Check sheet for the drawn part. Datum: minimum x, y, z corner. Units: mm. Give positions to 0.01 mm unless a question says otherwise; leave off trailing zeros. Loops run counter-clockwise (first coordinate to the right, second up) from the corner with the lowest first, then second, coordinate; pieces in that order, holes last.
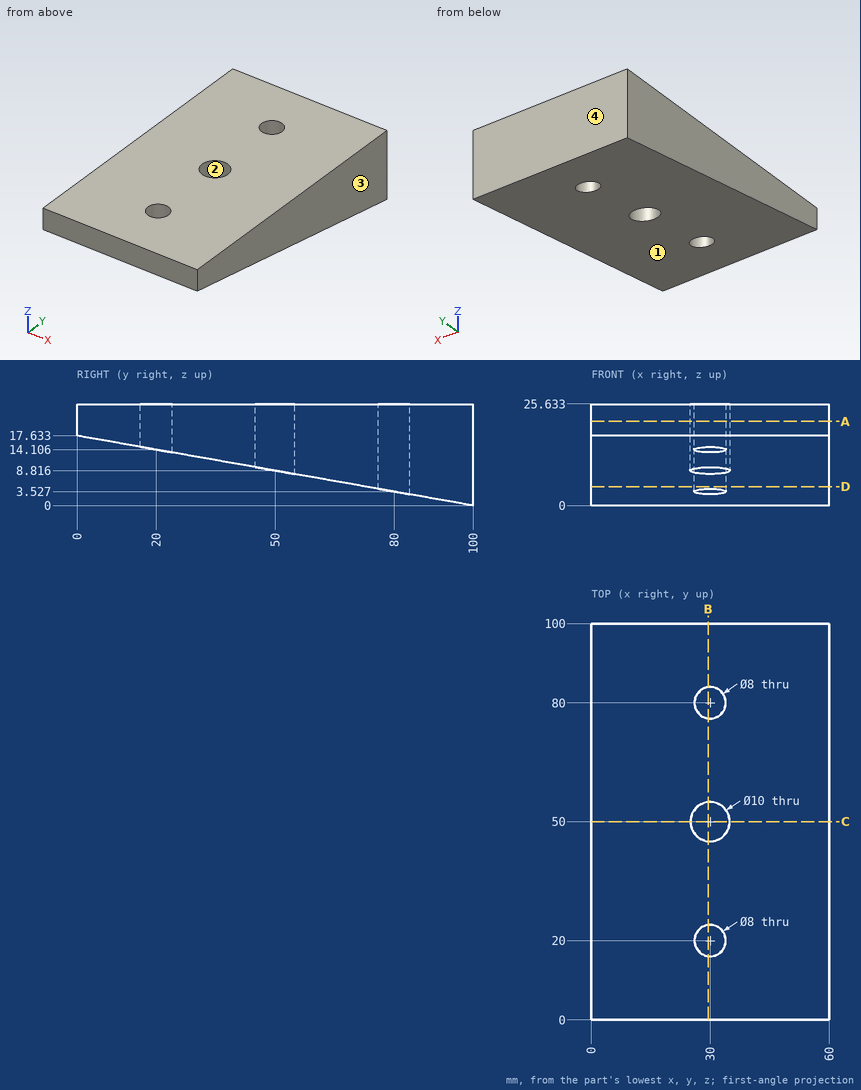
(1) Gauge pin test, flat ends, axial feed: pin 1 Ø4 at (x, y) = (11.5, 51) entering from -Z; pin 2 Ø2 at (x, y) = (20.5, 22) entering from -Z. Record the tip position at first contact, or that the pin passes through.
(2) Release check for a two-part mould opening along Y. For the marked faces 1, 2, 3 and 4 record: pulls with the +Y half, pulls with the -Y half, needs draft (parallel to the pull), parting line crosses it, or undercut.
(3) Material ranges on line 1 (Y direction, x = 30, z = 17.75); line 2 (X direction, y = 20, z = 19); line 3 (Y direction, x = 29, z = 24.5), recorded low to high.
(4) Section check B-B on x = 29.5. Record the boundary of the cut face in (y, z) (1 decimal), plus the area to 3 significant figures.
(5) Section check D-D on z = 4.75. Record the boundary of the cut face in (x, y).
(6) Section check A-A on z = 21.25. Record the boundary of the cut face in (x, y).
(7) Section check C-C on y = 50. Record the boundary of the cut face in (x, z), plus the area to 3 significant figures.
Computed values:
1. pin 1: stops at z = 8.29
1. pin 2: stops at z = 13.58
2. face 1: pulls with the -Y half
2. face 2: undercut
2. face 3: needs draft
2. face 4: pulls with the +Y half
3. line 1: y = 0 to 16, 24 to 45, 55 to 76, 84 to 100
3. line 2: x = 0 to 26, 34 to 60
3. line 3: y = 0 to 16.13, 23.87 to 45.1, 54.9 to 76.13, 83.87 to 100
4. outline: (0, 17.6) - (16, 14.8) - (16, 25.6) - (0, 25.6) - close; (24, 13.4) - (45, 9.7) - (45, 25.6) - (24, 25.6) - close; (55, 7.9) - (76, 4.2) - (76, 25.6) - (55, 25.6) - close; (84, 2.8) - (100, 0) - (100, 25.6) - (84, 25.6) - close
4. area: 1,250 mm2
5. outline: (0, 73.06) - (60, 73.06) - (60, 100) - (0, 100) - close; hole circle Ø8 at (30, 80)
6. outline: (0, 0) - (60, 0) - (60, 100) - (0, 100) - close; hole circle Ø10 at (30, 50); hole circle Ø8 at (30, 20); hole circle Ø8 at (30, 80)
7. outline: (0, 8.82) - (25, 8.82) - (25, 25.63) - (0, 25.63) - close; (35, 8.82) - (60, 8.82) - (60, 25.63) - (35, 25.63) - close
7. area: 841 mm2
